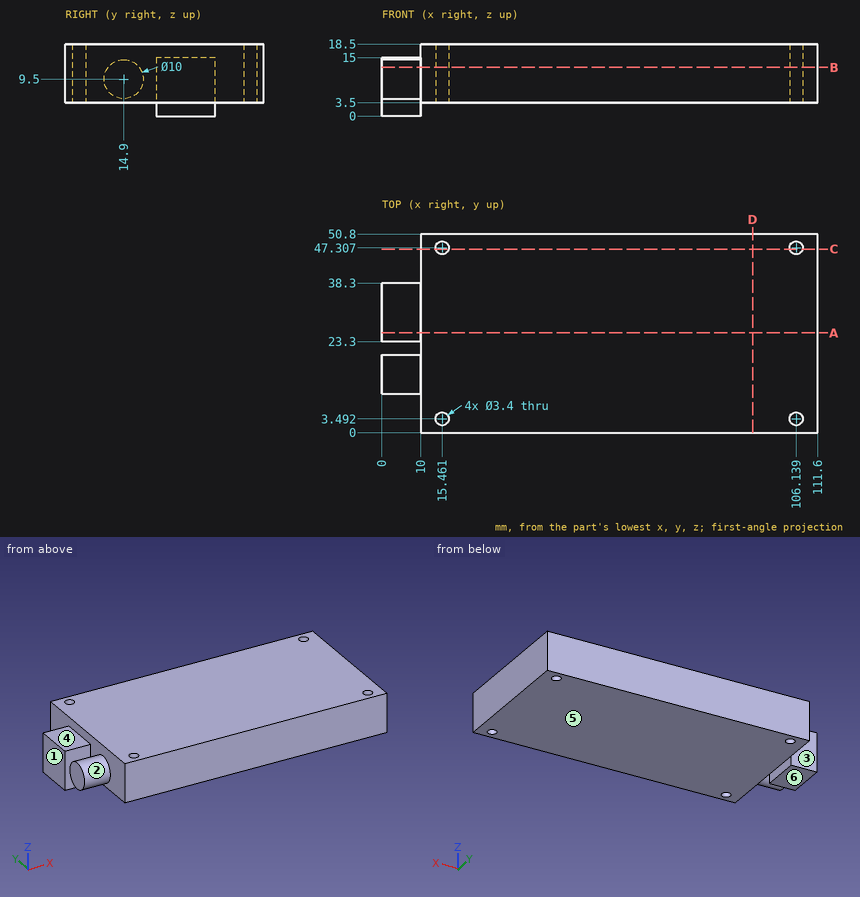
Input: dimensioned drawing with shaded views. Units: mm. Origin: part minimum x, y, z. A direction names the side the tool comes from. Give positions to 0.01 mm unless a question says otherwise; leave off trailing zeros. Order: outer loops, then holes, each group sorted by start corner. A loop starts at its lowest first (then second) coordinate and runs counter-clockwise, first axis right, second up. Notation, with made-up numbers: (-2.5, 66) -> (56.5, 66) arc R35 ccw to (56.5, 101) -> close; hole circle Ø8 at (57.5, 84.5). An arc over 180 degrees is marked (long way). Use one line per item in the form item = value.
1) Section B-B, the plane z = 12.5. Return loops of the section in (x, y).
Response values:
outline = (0, 10.9) -> (10, 10.9) -> (10, 0) -> (111.6, 0) -> (111.6, 50.8) -> (10, 50.8) -> (10, 38.3) -> (0, 38.3) -> (0, 23.3) -> (10, 23.3) -> (10, 18.9) -> (0, 18.9) -> close; hole circle Ø3.4 at (15.46, 3.49); hole circle Ø3.4 at (15.46, 47.31); hole circle Ø3.4 at (106.14, 3.49); hole circle Ø3.4 at (106.14, 47.31)
2) Line query: probe 1 along X at (y, z) = (6, 12.25); probe 2 along Z at (x, y) = (24, 23.5); probe 3 along Y at (x, z) = (7, 1.25). Output: solid intervals per line, ascending.
Response values:
probe_1 = 10 to 111.6
probe_2 = 3.5 to 18.5
probe_3 = 23.3 to 38.3
3) Section A-A, the plane y = 25.5. Return loops of the section in (x, z), and give its area (3 significant figures).
Response values:
outline = (0, 0) -> (10, 0) -> (10, 3.5) -> (111.6, 3.5) -> (111.6, 18.5) -> (10, 18.5) -> (10, 15) -> (0, 15) -> close
area = 1,670 mm^2
4) Section D-D, the plane x = 95. Return loops of the section in (y, z), and give its area (3 significant figures).
Response values:
outline = (0, 3.5) -> (50.8, 3.5) -> (50.8, 18.5) -> (0, 18.5) -> close
area = 762 mm^2
5) First-contact query: pin 1 Ø4.5 at (x, y) = (15.46, 47.31) entering from -Z; pin 2 Ø11 at (x, z) = (4, 8) entering from -Y; pin 3 Ø1 at (y, z) = (31, 2) entering from +X. Flat tips, straight axial feed; report the tip coordinate or a pass-through.
Response values:
pin_1 = 3.5
pin_2 = 9.9
pin_3 = 10
6) Section C-C, the plane y = 47. Return loops of the section in (x, z).
Response values:
outline = (10, 3.5) -> (13.79, 3.5) -> (13.79, 18.5) -> (10, 18.5) -> close; (17.13, 3.5) -> (104.47, 3.5) -> (104.47, 18.5) -> (17.13, 18.5) -> close; (107.81, 3.5) -> (111.6, 3.5) -> (111.6, 18.5) -> (107.81, 18.5) -> close
7) Mould query, pull axis Y, two halves, no side actions, for the marked faces 1, 2 and 3. Classes: pulls with the +Y half, pulls with the -Y half, needs draft (parallel to the pull), parting line crosses it, or undercut.
Response values:
face_1 = needs draft
face_2 = undercut
face_3 = pulls with the +Y half
8) Reachability of the marked faces 4, 5 and 6 from +Z, -Z, +X, -X, +Y, -Y: full face, straight path, thin tool, end or side. Return the list, or none.
Response values:
face_4 = +Z, -X, +Y, -Y
face_5 = -Z, +X, +Y, -Y
face_6 = -Z, +X, -X, +Y, -Y
